```python
from build123d import *

# Parameters (mm, degrees)
SKETCH4_W           = 32
SKETCH4_H           = 23
BOSS_EXTRUDE3_DEPTH = 9.5
SKETCH5_W           = 29
SKETCH5_H           = 20
CUT_EXTRUDE2_DEPTH  = 8
SKETCH7_W           = 10
SKETCH7_H           = 7
CUT_EXTRUDE4_DEPTH  = 36.305806888
BOSS_EXTRUDE4_DEPTH = 10
CUT_EXTRUDE5_DEPTH  = 5
SKETCH10_W          = 14
SKETCH10_H          = 3
CUT_EXTRUDE6_DEPTH  = 7.9
CIRPATTERN1_COUNT   = 2
SKETCH11_R          = 2.6
CUT_EXTRUDE7_DEPTH  = 7
CIRPATTERN2_COUNT   = 2
CUT_EXTRUDE8_REACH  = 26.739
SKETCH12_R          = 1.7
CUT_EXTRUDE9_START  = -10
SKETCH13_R          = 1.7
CUT_EXTRUDE9_DEPTH  = 10


with BuildPart() as part:
    # Sketch4 → Boss-Extrude3 (new body)
    with BuildSketch(Plane(origin=(0, 0, 0), x_dir=(1, 0, 0), z_dir=(0, 1, 0))):
        Rectangle(SKETCH4_W, SKETCH4_H)
    extrude(amount=BOSS_EXTRUDE3_DEPTH)

    # Sketch5 → Cut-Extrude2 (cut)
    with BuildSketch(Plane(origin=(0, 9.5, 0), x_dir=(1, 0, 0), z_dir=(0, 1, 0))):
        Rectangle(SKETCH5_W, SKETCH5_H)
    extrude(amount=-CUT_EXTRUDE2_DEPTH, mode=Mode.SUBTRACT)

    # Sketch7 → Cut-Extrude4 (cut, through all)
    with BuildSketch(Plane(origin=(16, 0, 0), x_dir=(0, 0, -1), z_dir=(1, 0, 0))):
        with Locations((0, 6)):
            Rectangle(SKETCH7_W, SKETCH7_H)
    extrude(amount=-CUT_EXTRUDE4_DEPTH, mode=Mode.SUBTRACT)

    # Sketch8 → Boss-Extrude4 (add)
    with BuildSketch(Plane(origin=(0, 0, 0), x_dir=(-1, 0, 0), z_dir=(0, -1, 0))):
        Polygon((-16, -9.5), (-1, -9.5), (-1, -11.5), (16, -11.5), (16, 9.5), (1, 9.5), (1, 11.5), (-16, 11.5), align=None)
    extrude(amount=BOSS_EXTRUDE4_DEPTH)

    # Sketch9 → Cut-Extrude5 (cut)
    with BuildSketch(Plane(origin=(0, 0, -9.5), x_dir=(-1, 0, 0), z_dir=(0, 0, -1))):
        with BuildLine():
            Line((3.5, -4.1), (13.5, -4.1))
            ThreePointArc((13.5, -4.1), (14.4, -5), (13.5, -5.9))
            Line((13.5, -5.9), (3.5, -5.9))
            ThreePointArc((3.5, -5.9), (2.6, -5), (3.5, -4.1))
        make_face()
    cut_extrude5 = extrude(amount=-CUT_EXTRUDE5_DEPTH, mode=Mode.SUBTRACT)

    # Sketch10 → Cut-Extrude6 (cut)
    with BuildSketch(Plane(origin=(0, -10, 0), x_dir=(-1, 0, 0), z_dir=(0, -1, 0))):
        with Locations((-8, -4)):
            Rectangle(SKETCH10_W, SKETCH10_H)
        with Locations((8, 4)):
            Rectangle(SKETCH10_W, SKETCH10_H)
    extrude(amount=-CUT_EXTRUDE6_DEPTH, mode=Mode.SUBTRACT)

    # CirPattern1: Cut-Extrude5 ×2 about axis
    cirpattern1_axis = Axis((0, 0, 0), (0, -1, 0))
    for i in range(1, CIRPATTERN1_COUNT):
        add(cut_extrude5.rotate(cirpattern1_axis, i * 360 / CIRPATTERN1_COUNT), mode=Mode.SUBTRACT)

    # Sketch11 → Cut-Extrude7 (cut)
    with BuildSketch(Plane(origin=(0, 0, -11.5), x_dir=(-1, 0, 0), z_dir=(0, 0, -1))):
        with Locations((-12.5, -5)):
            Circle(SKETCH11_R)
        with Locations((-2.5, -5)):
            Circle(SKETCH11_R)
    cut_extrude7 = extrude(amount=-CUT_EXTRUDE7_DEPTH, mode=Mode.SUBTRACT)

    # CirPattern2: Cut-Extrude7 ×2 about axis
    cirpattern2_axis = Axis((0, 0, 0), (0, -1, 0))
    for i in range(1, CIRPATTERN2_COUNT):
        add(cut_extrude7.rotate(cirpattern2_axis, i * 360 / CIRPATTERN2_COUNT), mode=Mode.SUBTRACT)

    # Cut-Extrude8: up to this face of the body (flat: up to its plane)
    cut_extrude8_end = Plane(part.part.faces().sort_by_distance((-7.885932934, -6.28954084, -5.5))[0])
    # Sketch12 → Cut-Extrude8 (cut, up to the picked face)
    with BuildSketch(Plane.XY.offset(4.5), mode=Mode.PRIVATE) as cut_extrude8_sk1:
        with Locations((-2.5, -5)):
            Circle(SKETCH12_R)
    cut_extrude8_tool1 = split(extrude(cut_extrude8_sk1.sketch, amount=-CUT_EXTRUDE8_REACH, mode=Mode.PRIVATE), bisect_by=cut_extrude8_end, keep=Keep.BOTH, mode=Mode.PRIVATE)
    # Sketch12 → Cut-Extrude8 (cut, up to the picked face)
    with BuildSketch(Plane.XY.offset(4.5), mode=Mode.PRIVATE) as cut_extrude8_sk2:
        with Locations((-12.5, -5)):
            Circle(SKETCH12_R)
    cut_extrude8_tool2 = split(extrude(cut_extrude8_sk2.sketch, amount=-CUT_EXTRUDE8_REACH, mode=Mode.PRIVATE), bisect_by=cut_extrude8_end, keep=Keep.BOTH, mode=Mode.PRIVATE)
    add(cut_extrude8_tool1.solids().sort_by(Axis((-2.5, -5, 4.5), (0, 0, -1)))[0], mode=Mode.SUBTRACT)
    add(cut_extrude8_tool2.solids().sort_by(Axis((-12.5, -5, 4.5), (0, 0, -1)))[0], mode=Mode.SUBTRACT)

    # Sketch13 → Cut-Extrude9 (cut)
    with BuildSketch(Plane(origin=(0, 0, -4.5), x_dir=(-1, 0, 0), z_dir=(0, 0, -1)).offset(CUT_EXTRUDE9_START)):
        with Locations((-12.5, -5)):
            Circle(SKETCH13_R)
        with Locations((-2.5, -5)):
            Circle(SKETCH13_R)
    extrude(amount=CUT_EXTRUDE9_DEPTH, mode=Mode.SUBTRACT)


solid = part.part
```
Model file for the job. Use its own axes, mm. A direction names the side the tool comes from. Give positions to 0.01 mm unless a question says otherwise; leave off trailing zeros. Loops run counter-clockwise (first coordinate to the right, second up) from the corner with the lowest first, then second, coordinate; pieces in that order, holes last. Notation, with made-up numbers: (60.25, -3) - (108.25, -3) arc R25 ccw to (108.25, 28) - close; hole circle Ø9 at (-17, 28). An arc over 180 degrees is marked (long way). One line per item, written item: value. Start each with the question number.
1. Which spindle directions (+Z, -Z, +X, -X, +Y, -Y) get a long thin tool onto all of the face, cutting with end or side? Do faces 1 (the flat face through (14.5, 2, 0)), 2 (the cylindrical face through (-5.1, -4.9, 8)), 3 (the flat face through (-15, 6, 5)). Say none if no direction does.
2. Pin check, flat tips, straight feed: pin 1 (6.5 mm diameter, centred on x = -5, y = -7, fed in from -Z); pin 2 (1 mm diameter, centred on x = 12, z = 3, fed in from +Y); pin 3 (8 mm diameter, centred on x = 7, y = -6, fed in from +Z). Stop position of each tip, or through.
3. Slice it at B-B (y = 3). List the corners of the cut face in (x, z), plus the area to 3 significant figures.
4. Slice it at C-C (z = 6). List the corners of the cut face in (x, y).
5. Slice it at A-A (x = -12.5). List the corners of the cut face in (y, z).
6. Probe L1, parallel to Z at x = 1.5, y = 3; L2, parallel to Y at x = -8, z = -7; L3, parallel to Z at x = 6, y = -4. List the from-to ranges inside material, lowest first. Write a range as from..to.
7. Pull direction Z, two halves, no side cores. Call faces 4 (the flat face through (8.6, -3.8, 9.5)), 5 (the flat face through (-0.1, 9.5, 10.2)), 6 (the flat face through (15, 2.5, 0)): pulls with the +Z half, pulls with the -Z half, needs draft (parallel to the pull), parting line crosses it, or undercut.
8. Slice it at D-D (x = 7.5). List the corners of the cut face in (y, z), plus the area to 3 significant figures.
Solution:
1. face 1: +Y
1. face 2: +Z
1. face 3: +X, -X, +Y
2. pin 1: stops at z = -9.5
2. pin 2: stops at y = 1.5
2. pin 3: stops at z = 9.5
3. outline: (-16, -11.5) - (16, -11.5) - (16, -5) - (14.5, -5) - (14.5, -10) - (-14.5, -10) - (-14.5, -5) - (-16, -5) - close; (-16, 5) - (-14.5, 5) - (-14.5, 10) - (14.5, 10) - (14.5, 5) - (16, 5) - (16, 11.5) - (-16, 11.5) - close
3. area: 126 mm^2
4. outline: (-16, -10) - (16, -10) - (16, 9.5) - (14.5, 9.5) - (14.5, 1.5) - (-14.5, 1.5) - (-14.5, 9.5) - (-16, 9.5) - close; hole circle Ø5.2 at (-12.5, -5); hole circle Ø5.2 at (-2.5, -5); hole (3.5, -5.9) - (13.5, -5.9) arc R0.9 ccw to (13.5, -4.1) - (3.5, -4.1) arc R0.9 ccw to start
5. outline: (-10, -9.5) - (-5.9, -9.5) - (-5.9, -5.5) - (-10, -5.5) - close; (-10, -2.5) - (-6.7, -2.5) - (-6.7, 4.5) - (-7.6, 4.5) - (-7.6, 11.5) - (-10, 11.5) - close; (-4.1, -9.5) - (0, -9.5) - (0, -11.5) - (9.5, -11.5) - (9.5, -10) - (1.5, -10) - (1.5, 10) - (9.5, 10) - (9.5, 11.5) - (-2.4, 11.5) - (-2.4, 4.5) - (-3.3, 4.5) - (-3.3, -2.5) - (-2.1, -2.5) - (-2.1, -5.5) - (-4.1, -5.5) - close
6. L1: z = -11.5..-10, 10..11.5
6. L2: y = -10..-5.9, -4.1..1.5
6. L3: z = -11.5..2.5, 5.5..9.5
7. face 4: pulls with the +Z half
7. face 5: needs draft
7. face 6: undercut
8. outline: (-10, -11.5) - (9.5, -11.5) - (9.5, -10) - (1.5, -10) - (1.5, 10) - (9.5, 10) - (9.5, 11.5) - (0, 11.5) - (0, 9.5) - (-4.1, 9.5) - (-4.1, 5.5) - (-2.1, 5.5) - (-2.1, 2.5) - (-10, 2.5) - close; (-10, 5.5) - (-5.9, 5.5) - (-5.9, 9.5) - (-10, 9.5) - close
8. area: 238 mm^2
